For this review, take the finished solid that the model builds, in its own axes (mm). A direction names the side the tool comes from. Give positions to 0.01 mm unless a question says otherwise; leave off trailing zeros. Order: outer loops, then holes, each group sorted by start corner. A loop starts at its lowest first (then second) coordinate and runs counter-clockwise, first axis right, second up.
from build123d import *

# Parameters (mm, degrees)
SKETCH1_W           = 200
SKETCH1_H           = 110
BOSS_EXTRUDE1_DEPTH = 5
SKETCH4_R           = 1.5
CUT_EXTRUDE1_DEPTH  = 10
BOSS_EXTRUDE2_DEPTH = 20
SKETCH7_W           = 43.6
SKETCH7_H           = 43.6
BOSS_EXTRUDE3_DEPTH = 3
SKETCH7_3_W         = 49.6
SKETCH7_3_H         = 49.6
SKETCH7_3_W_2       = 43.6
SKETCH7_3_H_2       = 43.6
BOSS_EXTRUDE4_DEPTH = 5
SKETCH8_W           = 87.6
SKETCH8_H           = 58.6
SKETCH8_W_2         = 83.6
SKETCH8_H_2         = 54.6
BOSS_EXTRUDE5_DEPTH = 4
SKETCH9_R           = 1.5
CUT_EXTRUDE2_DEPTH  = 5


with BuildPart() as part:
    # Sketch1 → Boss-Extrude1 (new body)
    with BuildSketch(Plane(origin=(0, 0, 0), x_dir=(1, 0, 0), z_dir=(0, 1, 0))):
        Rectangle(SKETCH1_W, SKETCH1_H)
    extrude(amount=BOSS_EXTRUDE1_DEPTH)

    # Sketch4 → Cut-Extrude1 (cut)
    with BuildSketch(Plane(origin=(0, 5, 0), x_dir=(1, 0, 0), z_dir=(0, 1, 0))):
        with Locations(Location((94.5, 49.5, 0), (0, 0, 270))):
            Circle(SKETCH4_R)
        with Locations(Location((-94.5, 49.5, 0), (0, 0, 270))):
            Circle(SKETCH4_R)
        with Locations(Location((-94.5, -49.5, 0), (0, 0, 270))):
            Circle(SKETCH4_R)
        with Locations(Location((94.5, -49.5, 0), (0, 0, 270))):
            Circle(SKETCH4_R)
    extrude(amount=-CUT_EXTRUDE1_DEPTH, mode=Mode.SUBTRACT)

    # Sketch5 → Boss-Extrude2 (add)
    with BuildSketch(Plane(origin=(0, 5, 0), x_dir=(1, 0, 0), z_dir=(0, 1, 0))):
        Polygon((85, -19.9), (85, -45), (-9.1, -45), (-9.1, -19.9), (-11.1, -19.9), (-11.1, -47), (87, -47), (87, -17.9), (72, -17.9), (72, -19.9), align=None)
    extrude(amount=BOSS_EXTRUDE2_DEPTH)

    # Sketch7 → Boss-Extrude3 (add)
    with BuildSketch(Plane(origin=(0, 5, 0), x_dir=(1, 0, 0), z_dir=(0, 1, 0))):
        with Locations((63.2, 17.9)):
            Rectangle(SKETCH7_W, SKETCH7_H)
    extrude(amount=BOSS_EXTRUDE3_DEPTH)

    # Sketch7_3 → Boss-Extrude4 (add)
    with BuildSketch(Plane(origin=(0, 5, 0), x_dir=(1, 0, 0), z_dir=(0, 1, 0))):
        with Locations((63.2, 17.9)):
            Rectangle(SKETCH7_3_W, SKETCH7_3_H)
        with Locations((63.2, 17.9)):
            Rectangle(SKETCH7_3_W_2, SKETCH7_3_H_2, mode=Mode.SUBTRACT)
    extrude(amount=BOSS_EXTRUDE4_DEPTH)

    # Sketch8 → Boss-Extrude5 (add)
    with BuildSketch(Plane(origin=(0, 5, 0), x_dir=(1, 0, 0), z_dir=(0, 1, 0))):
        with Locations((-15.4, 17.4)):
            Rectangle(SKETCH8_W, SKETCH8_H)
        with Locations((-15.4, 17.4)):
            Rectangle(SKETCH8_W_2, SKETCH8_H_2, mode=Mode.SUBTRACT)
    extrude(amount=BOSS_EXTRUDE5_DEPTH)

    # Sketch9 → Cut-Extrude2 (cut)
    with BuildSketch(Plane(origin=(0, 5, 0), x_dir=(1, 0, 0), z_dir=(0, 1, 0))):
        with Locations(Location((-18.6, -49.5, 0), (0, 0, 270))):
            Circle(SKETCH9_R)
        with Locations(Location((-18.6, 49.5, 0), (0, 0, 270))):
            Circle(SKETCH9_R)
    extrude(amount=-CUT_EXTRUDE2_DEPTH, mode=Mode.SUBTRACT)


solid = part.part
1) Tool access review of faces 4 (the face through (-19, 9, 11)), 5 (the face through (63, 7, -42.7)), 6 (the face through (87, 15, 33)), 7 (the face through (-16, 7, 9.9)), 8 (the face through (-16, 7, 11.9)): name each direction out of +Z, -Z, +X, -X, +Y, -Y from which nothing blocks a thin tool from reaching the whole face with its end or side.
Answer sheet:
face 4: -Z, -X, +Y
face 5: -Z, +X, +Y
face 6: +Z, +X, +Y
face 7: +Y
face 8: +X, -X, +Y
2) Draft analysis for pull direction X (two halves, no side actions). For faces 1 (the face through (88, 7, -18)), 2 (the face through (39, 15, 45)), 3 (the face through (37, 15, 47)), state which applies: +X half, -X half, draft (parallel to the pull), parting line (faces both ways), or undercut.
Answer sheet:
face 1: +X half
face 2: undercut
face 3: draft
3) We need section D-D on z = -11. Give the boundary of the cut face in (x, y), then the cut area to 3 significant figures.
Answer sheet:
outline: (-100, 0) - (100, 0) - (100, 5) - (88, 5) - (88, 10) - (85, 10) - (85, 8) - (41.4, 8) - (41.4, 10) - (38.4, 10) - (38.4, 5) - (28.4, 5) - (28.4, 9) - (26.4, 9) - (26.4, 5) - (-57.2, 5) - (-57.2, 9) - (-59.2, 9) - (-59.2, 5) - (-100, 5) - close
area: 1,180 mm2
4) We need section A-A on y = 20.75. Give the boundary of the cut face in (x, z), then the cut area to 3 significant figures.
Answer sheet:
outline: (-11.1, 19.9) - (-9.1, 19.9) - (-9.1, 45) - (85, 45) - (85, 19.9) - (72, 19.9) - (72, 17.9) - (87, 17.9) - (87, 47) - (-11.1, 47) - close
area: 327 mm2
5) To check wall thickness, follow line 1 (Z direction, x = -94.5, y = 2.85); line 2 (X direction, y = 1.7, z = -49.5); line 3 (Z direction, x = 76.5, y = 9.5). State the ranges of each line that lie inside material, in increasing order.
Answer sheet:
line 1: z = -55 to -51, -48 to 48, 51 to 55
line 2: x = -100 to -96, -93 to -20.1, -17.1 to 93, 96 to 100
line 3: z = -42.7 to -39.7, 3.9 to 6.9, 17.9 to 19.9, 45 to 47
6) We need section B-B on x = 48.5. Give the boundary of the cut face in (y, z).
Answer sheet:
outline: (0, -55) - (5, -55) - (5, -42.7) - (10, -42.7) - (10, -39.7) - (8, -39.7) - (8, 3.9) - (10, 3.9) - (10, 6.9) - (5, 6.9) - (5, 45) - (25, 45) - (25, 47) - (5, 47) - (5, 55) - (0, 55) - close
7) Clearance check with flat-ended pins moving along their axes: pin 1 (2.5 mm diameter, centred on y = 8, z = -19, fed in from +X); pin 2 (1 mm diameter, centred on x = -10.5, y = 19.5, fed in from -Z); pin 3 (1.6 mm diameter, centred on y = 16.5, z = 19, fed in from -X); pin 4 (2 mm diameter, centred on x = -30.5, z = -29.5, fed in from -Y). State where each tip first meets the part, or that it passes through.
Answer sheet:
pin 1: stops at x = 88
pin 2: stops at z = 19.9
pin 3: stops at x = 72
pin 4: stops at y = 0
8) We need section C-C on z = 24.5. Give the boundary of the cut face in (x, y), then the cut area to 3 significant figures.
Answer sheet:
outline: (-100, 0) - (100, 0) - (100, 5) - (87, 5) - (87, 25) - (85, 25) - (85, 5) - (-9.1, 5) - (-9.1, 25) - (-11.1, 25) - (-11.1, 5) - (-100, 5) - close
area: 1,080 mm2
